from build123d import *

# Parameters (mm, degrees)
CUT_EXTRUDE_1_DEPTH = 8.918334965


with BuildPart() as part:
    # 草图1 → 旋转2 (revolve)
    with BuildSketch(Plane.XY):
        with BuildLine():
            Line((-2.925029572, 5.6), (-4.925029572, 5.6))
            Line((-4.925029572, 5.6), (-4.925029572, 9.366722189))
            Line((-4.925029572, 9.366722189), (-2.925029572, 9.366722189))
            ThreePointArc((-2.925029572, 9.366722189), (-1.636083126, 8.287220203), (0, 7.9))
            Line((0, 7.9), (0, 6.6))
            ThreePointArc((0, 6.6), (-1.54562269, 6.343093076), (-2.925029572, 5.6))
        make_face()
    revolve(axis=Axis((0, 7.9, 0), (0, -1, 0)))

    # 草图2 → 切除-拉伸1 (cut, through all)
    with BuildSketch(Plane(origin=(0, 9.366722189, 0), x_dir=(1, 0, 0), z_dir=(0, 1, 0))):
        with BuildLine():
            Line((-0.347296355, 1.969615506), (-1.736481777, 9.84807753))
            ThreePointArc((-1.736481777, 9.84807753), (0, 10), (1.736481777, 9.84807753))
            Line((1.736481777, 9.84807753), (0.347296355, 1.969615506))
            ThreePointArc((0.347296355, 1.969615506), (0, 2), (-0.347296355, 1.969615506))
        make_face()
        with BuildLine():
            Line((1.879385242, -0.684040287), (9.396926208, -3.420201433))
            ThreePointArc((9.396926208, -3.420201433), (8.660254038, -5), (7.660444431, -6.427876097))
            Line((7.660444431, -6.427876097), (1.532088886, -1.285575219))
            ThreePointArc((1.532088886, -1.285575219), (1.732050808, -1), (1.879385242, -0.684040287))
        make_face()
        with BuildLine():
            Line((-1.532088886, -1.285575219), (-7.660444431, -6.427876097))
            ThreePointArc((-7.660444431, -6.427876097), (-8.660254038, -5), (-9.396926208, -3.420201433))
            Line((-9.396926208, -3.420201433), (-1.879385242, -0.684040287))
            ThreePointArc((-1.879385242, -0.684040287), (-1.732050808, -1), (-1.532088886, -1.285575219))
        make_face()
    extrude(amount=-CUT_EXTRUDE_1_DEPTH, mode=Mode.SUBTRACT)


solid = part.part
Verification items for the finished model (mm, model axes). A direction names the side the tool comes from. Give positions to 0.01 mm unless a question says otherwise; leave off trailing zeros. Write each loop counter-clockwise with the first axis right and the second up, starting at its lowest first coordinate (ties: lowest second). Pieces come first, ordered by that corner, then holes. Notation, with made-up numbers: M -30,52.5 L -17,52.5 A14 ccw -17,65.5 Z; hole C 72,63 d10. An arc over 180 degrees is marked long. Put each result on its own line as item: value. Start each with the question number.
1. Scan lines: line 1 along X through (y, z) = (6.05, -3.5); line 2 along Z through (x, y) = (2, 6.8); line 3 along Z through (x, y) = (-3.25, 8.6). Record each from-to range of solid material in increasing order. Write a range as [from, to].
2. Section check A-A (z = -2.25). Record the cut outline in (x, y), and give its area (3 significant figures).
3. Section check C-C (y = 7.1). Record the cut outline in (x, z), and give its area (3 significant figures).
4. Section check D-D (y = 8.85). Record the cut outline in (x, z).
5. Section check B-B (x = -2). Record the cut outline in (y, z), and give its area (3 significant figures).
6. Draft check along X on faces 4 (the face through (3, 5.6, -2)), 5 (the face through (3.234, 7.51, 1.177)), 6 (the face through (4.235, 7.51, -2.514)), 7 (the face through (0.6, 7.5, -3.4)). Enter one of: +X half, -X half, draft (parallel to the pull), parting line (faces both ways), or undercut.
7. Set-up check for faces 1 (the face through (-0.6, 7.5, -3.4)), 2 (the face through (-2.637, 7.51, 2.213)), 3 (the face through (-3, 9.367, -2)): record each of +Z, -Z, +X, -X, +Y, -Y from which the full face is reachable in a straight line by a thin tool's end or side.
Answer list:
1. line 1: [-3.46, -0.62], [0.62, 3.46]
1. line 2: [-4.5, 0.73], [1.68, 4.5]
1. line 3: [-3.7, 1.18], [2.73, 3.7]
2. outline: M -4.38,5.6 L -1.87,5.6 A4.21 cw -0.4,6.02 L -0.4,8.7 A2.87 cw -1.87,9.37 L -4.38,9.37 Z; M 0.4,6.02 A4.21 cw 1.87,5.6 L 4.38,5.6 L 4.38,9.37 L 1.87,9.37 A2.87 cw 0.4,8.7 Z
2. area: 28.0 mm2
3. outline: M -4.63,1.68 A4.93 ccw -0.86,-4.85 L -0.35,-1.97 A2 ccw 0.35,-1.97 L 0.86,-4.85 A4.93 ccw 4.63,1.68 L 1.88,0.68 A2 ccw 1.53,1.29 L 3.77,3.17 A4.93 ccw -3.77,3.17 L -1.53,1.29 A2 ccw -1.88,0.68 Z
3. area: 65.6 mm2
4. outline: M -4.63,1.68 A4.93 ccw -0.86,-4.85 L -0.43,-2.42 A2.46 cw -2.31,0.84 Z; M -3.77,3.17 L -1.88,1.58 A2.46 cw 1.88,1.58 L 3.77,3.17 A4.93 ccw Z; M 0.43,-2.42 L 0.86,-4.85 A4.93 ccw 4.63,1.68 L 2.31,0.84 A2.46 cw Z
5. outline: M 5.6,-4.5 L 9.37,-4.5 L 9.37,-2.13 A3.05 cw 8.58,0.73 L 6.1,0.73 A4.34 cw 5.6,-2.13 Z; M 5.6,2.13 A4.34 cw 5.82,1.68 L 9,1.68 A3.05 cw 9.37,2.13 L 9.37,4.5 L 5.6,4.5 Z
5. area: 27.1 mm2
6. face 4: draft
6. face 5: undercut
6. face 6: +X half
6. face 7: undercut
7. face 1: -Z, +Y, -Y
7. face 2: +Y, -Y
7. face 3: +Z, -Z, +X, -X, +Y
